For this review, use the dimensioned drawing (mm, ordinates from the lowest corner) and the shaded views. A direction names the side the tool comes from. Give positions to 0.01 mm unless a question says otherwise; leave off trailing zeros. Order: outer loops, then holes, each group sorted by start corner. A loop starts at its lowest first (then second) coordinate and runs counter-clockwise, first axis right, second up.
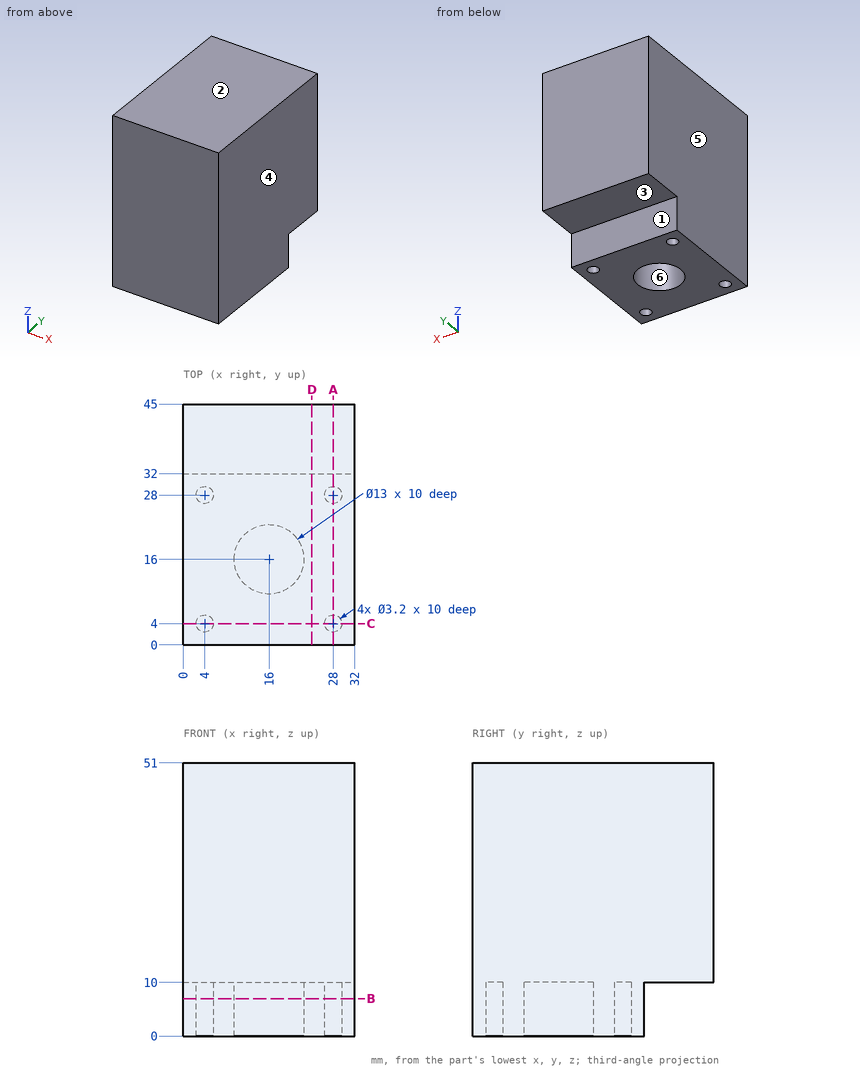
1. For the marked faces 1 and 2, list the 3-axis set-ups (+Z, -Z, +X, -X, +Y, -Y) from which the entire face can be reached by the end or side of a thin tool; tool diameter is ignored.
2. Take a section at D-D (x = 24). Write out the cut boundary in (y, z), and give its area (4 significant figures).
3. To check wall thickness, follow line 1 (Y direction, x = 4, z = 7.75); line 2 (Y direction, x = 16, z = 6.25); line 3 (Z direction, x = 20.5, y = 41.5). State the ranges of each line that lie inside material, in increasing order.
4. Draft analysis for pull direction X (two halves, no side actions). For the marked faces 3, 4, 5 and 6, state which applies: pulls with the +X half, pulls with the -X half, needs draft (parallel to the pull), parting line crosses it, or undercut.
5. Take a section at C-C (y = 4). Write out the cut boundary in (x, z).
6. Take a section at B-B (z = 7). Write out the cut boundary in (x, y).
7. Take a section at A-A (x = 28). Write out the cut boundary in (y, z), and give its area (3 significant figures).
8. Insertion check: pin 1 (4 mm diameter, centred on x = 17.5, y = 41.5, fed in from -Z); pin 2 (3 mm diameter, centred on x = 14, z = 3.5, fed in from +Y). Each pin has a flat end and moves straight along its axis. Give the tip position at first contact, or say it passes through.
Answer:
1. face 1: -Z, +X, -X, +Y
1. face 2: +Z, +X, -X, +Y, -Y
2. outline: (0, 0) - (32, 0) - (32, 10) - (45, 10) - (45, 51) - (0, 51) - close
2. area: 2,165 mm2
3. line 1: y = 0 to 2.4, 5.6 to 26.4, 29.6 to 32
3. line 2: y = 0 to 9.5, 22.5 to 32
3. line 3: z = 10 to 51
4. face 3: needs draft
4. face 4: pulls with the +X half
4. face 5: pulls with the -X half
4. face 6: undercut
5. outline: (0, 0) - (2.4, 0) - (2.4, 10) - (5.6, 10) - (5.6, 0) - (26.4, 0) - (26.4, 10) - (29.6, 10) - (29.6, 0) - (32, 0) - (32, 51) - (0, 51) - close
6. outline: (0, 0) - (32, 0) - (32, 32) - (0, 32) - close; hole circle Ø3.2 at (4, 4); hole circle Ø3.2 at (4, 28); hole circle Ø13 at (16, 16); hole circle Ø3.2 at (28, 4); hole circle Ø3.2 at (28, 28)
7. outline: (0, 0) - (2.4, 0) - (2.4, 10) - (5.6, 10) - (5.6, 0) - (26.4, 0) - (26.4, 10) - (29.6, 10) - (29.6, 0) - (32, 0) - (32, 10) - (45, 10) - (45, 51) - (0, 51) - close
7. area: 2,100 mm2
8. pin 1: stops at z = 10
8. pin 2: stops at y = 32
